Here's how the part is built. I have some questions about the finished solid (model axes, mm). A direction names the side the tool comes from. Round coordinates to 2 decimals unless told otherwise and drop trailing zeros. Order: outer loops, then holes, each group sorted by start corner. A loop starts at its lowest first (then second) coordinate and runs counter-clockwise, first axis right, second up. Notation, with made-up numbers: (8.5, 69) -> (62.5, 69) arc R21 cw to (62.5, 83) -> close; hole circle Ø8 at (41, -11). An arc over 180 degrees is marked (long way). Use a Markdown table: item, result. Add a question column.
(1) I'm going to push flat-ended pins straight in: P1, Ø1, axis at x = 17.5, z = 2, coming from the +Y side; P2, Ø1, axis at y = -18.5, z = 3, coming from the +X side. Where does each tip first touch, or does it pass through?
(2) On a 3-axis mill with a long thin cutter (end or side, diameter ignored), from which of +Z, -Z, +X, -X, +Y, -Y can I reach the whole of each face in a straight line? I mean faces 5 (the face through (-1.99, -24.17, 1.97)), 6 (the face through (17.656, -16.623, 1.972)), 7 (the face through (-23.12, 7.32, 1.97)), 8 (the face through (12.277, 20.912, 1.972)). Say none if no direction works.
(3) I want a section at B-B, the plane x = 0. Please give me the cut outline in (y, z), then the cut area to 3 significant figures.
(4) Thinking about a two-plate mould opening in Y: for faces 1 (the face through (5.07, 24.48, 1.97)), 2 (the face through (20.07, -13.57, 1.97)), 3 (the face through (-17.698, -16.551, 1.972)), 4 (the face through (10.167, -21.187, 1.972)), which applies, pulls with the +Y half, pulls with the -Y half, needs draft (parallel to the pull), parting line crosses it, or undercut?
(5) I want a section at A-A, the plane y = 0. Please give me the cut outline in (x, z), then the cut area to 3 significant figures.
(6) If I drill on probe 1 along Y at (x, z) = (0, 1.85); probe 2 along X at (y, z) = (-11, 2.25); probe 3 along Y at (x, z) = (-11, 3.05), over which ranges is the centre line in solid material (lowest first)?
from build123d import *

# Parameters (mm, degrees)
SKETCH1_R           = 16
BOSS_EXTRUDE1_DEPTH = 4


with BuildPart() as part:
    # Sketch1 → Boss-Extrude1 (new body)
    with BuildSketch(Plane.XY):
        with BuildLine():
            Line((24.836944886, 2.850643567), (23.14914702, 4.045613953))
            ThreePointArc((23.14914702, 4.045613953), (22.909534515, 5.234809289), (22.60887418, 6.410055249))
            Line((22.60887418, 6.410055249), (23.658232882, 8.080100055))
            ThreePointArc((23.658232882, 8.080100055), (22.276156802, 11.347812041), (20.445418397, 14.386968637))
            ThreePointArc((20.445418397, 14.386968637), (18.373039838, 14.652010344), (18.575790893, 16.731407374))
            ThreePointArc((18.575790893, 16.731407374), (16.072080469, 19.149105186), (13.25685896, 21.195652633))
            Line((13.25685896, 21.195652633), (11.270268735, 20.621130974))
            ThreePointArc((11.270268735, 20.621130974), (10.191122428, 21.175245539), (9.084819485, 21.672933694))
            Line((9.084819485, 21.672933694), (8.433390327, 23.534611269))
            ThreePointArc((8.433390327, 23.534611269), (5.01687988, 24.491445778), (1.499324848, 24.955))
            ThreePointArc((1.499324848, 24.955), (0, 23.5), (-1.499324848, 24.955))
            ThreePointArc((-1.499324848, 24.955), (-4.950595028, 24.504930297), (-8.305912153, 23.579902954))
            Line((-8.305912153, 23.579902954), (-9.095351779, 21.668515778))
            ThreePointArc((-9.095351779, 21.668515778), (-10.201412708, 21.170290002), (-11.280289579, 20.615651021))
            Line((-11.280289579, 20.615651021), (-13.141967154, 21.267080179))
            ThreePointArc((-13.141967154, 21.267080179), (-16.020209918, 19.192521309), (-18.575790893, 16.731407374))
            ThreePointArc((-18.575790893, 16.731407374), (-18.373039838, 14.652010344), (-20.445418397, 14.386968637))
            ThreePointArc((-20.445418397, 14.386968637), (-22.245371495, 11.408043085), (-23.614162005, 8.208005408))
            Line((-23.614162005, 8.208005408), (-22.611986892, 6.399066244))
            ThreePointArc((-22.611986892, 6.399066244), (-22.912076004, 5.223674298), (-23.151110514, 4.034362646))
            Line((-23.151110514, 4.034362646), (-24.821155321, 2.985003945))
            ThreePointArc((-24.821155321, 2.985003945), (-24.993754895, -0.558763162), (-24.662957214, -4.091276263))
            ThreePointArc((-24.662957214, -4.091276263), (-22.910805936, -5.229241948), (-23.995694883, -7.014743551))
            ThreePointArc((-23.995694883, -7.014743551), (-22.788929503, -10.279333251), (-21.140466226, -13.344687622))
            Line((-21.140466226, -13.344687622), (-19.101334675, -13.689010689))
            ThreePointArc((-19.101334675, -13.689010689), (-18.369478748, -14.656474696), (-17.588673036, -15.584883087))
            Line((-17.588673036, -15.584883087), (-17.809507272, -17.544841143))
            ThreePointArc((-17.809507272, -17.544841143), (-15.146492656, -19.889287575), (-12.178413721, -21.833145427))
            ThreePointArc((-12.178413721, -21.833145427), (-10.196267869, -21.172768396), (-9.476723699, -23.13421077))
            ThreePointArc((-9.476723699, -23.13421077), (-6.171958786, -24.22616199), (-2.747568192, -24.848558691))
            Line((-2.747568192, -24.848558691), (-1.206987851, -23.468983368))
            ThreePointArc((-1.206987851, -23.468983368), (0.005710674, -23.499999306), (1.218393982, -23.468393982))
            Line((1.218393982, -23.468393982), (2.613063, -24.863063))
            ThreePointArc((2.613063, -24.863063), (6.106387485, -24.242772776), (9.476723699, -23.13421077))
            ThreePointArc((9.476723699, -23.13421077), (10.196267869, -21.172768396), (12.178413721, -21.833145427))
            ThreePointArc((12.178413721, -21.833145427), (15.092622782, -19.930196626), (17.714304731, -17.640958247))
            Line((17.714304731, -17.640958247), (17.596245443, -15.576332891))
            ThreePointArc((17.596245443, -15.576332891), (18.376599843, -14.647545126), (19.107985481, -13.679725541))
            Line((19.107985481, -13.679725541), (21.067943537, -13.458891304))
            ThreePointArc((21.067943537, -13.458891304), (22.761033302, -10.340955615), (23.995694883, -7.014743551))
            ThreePointArc((23.995694883, -7.014743551), (22.910805936, -5.229241948), (24.662957214, -4.091276263))
            ThreePointArc((24.662957214, -4.091276263), (24.992151562, -0.626386701), (24.836944886, 2.850643567))
        make_face()
        Circle(SKETCH1_R, mode=Mode.SUBTRACT)
    extrude(amount=BOSS_EXTRUDE1_DEPTH)


solid = part.part
Taken from the geometry:
| question | item | result |
|---|---|---|
| 1 | P1 | stops at y = 18.33 |
| 1 | P2 | stops at x = 17.35 |
| 2 | face 5 | +Z, -Z, -Y |
| 2 | face 6 | +Z, -Z, +X |
| 2 | face 7 | +Z, -Z, -X |
| 2 | face 8 | +Z, -Z, +Y |
| 3 | outline | (-23.5, 0) -> (-16, 0) -> (-16, 4) -> (-23.5, 4) -> close; (16, 0) -> (23.5, 0) -> (23.5, 4) -> (16, 4) -> close |
| 3 | area | 60.0 mm2 |
| 4 | face 1 | pulls with the +Y half |
| 4 | face 2 | pulls with the -Y half |
| 4 | face 3 | undercut |
| 4 | face 4 | undercut |
| 5 | outline | (-25, 0) -> (-16, 0) -> (-16, 4) -> (-25, 4) -> close; (16, 0) -> (25, 0) -> (25, 4) -> (16, 4) -> close |
| 5 | area | 72.0 mm2 |
| 6 | probe 1 | y = -23.5 to -16, 16 to 23.5 |
| 6 | probe 2 | x = -22.45 to -11.62, 11.62 to 22.45 |
| 6 | probe 3 | y = -21.03 to -11.62, 11.62 to 20.77 |
